from build123d import *

# Parameters (mm, degrees)
SKETCH1_W           = 50
SKETCH1_H           = 32
SKETCH1_R           = 9.5
SKETCH1_R_2         = 1.65
BOSS_EXTRUDE1_DEPTH = 6.35
SKETCH2_R           = 1.65
CUT_EXTRUDE1_DEPTH  = 31.892110643
FILLET1_R           = 4


with BuildPart() as part:
    # Sketch1 → Boss-Extrude1 (new body)
    with BuildSketch(Plane.XY):
        with Locations((0, -1)):
            Rectangle(SKETCH1_W, SKETCH1_H)
        Circle(SKETCH1_R, mode=Mode.SUBTRACT)
        with Locations((-9.192388155, 9.192388155)):
            Circle(SKETCH1_R_2, mode=Mode.SUBTRACT)
        with Locations((9.192388155, 9.192388155)):
            Circle(SKETCH1_R_2, mode=Mode.SUBTRACT)
        with Locations((9.192388155, -9.192388155)):
            Circle(SKETCH1_R_2, mode=Mode.SUBTRACT)
        with Locations((-9.192388155, -9.192388155)):
            Circle(SKETCH1_R_2, mode=Mode.SUBTRACT)
    extrude(amount=BOSS_EXTRUDE1_DEPTH)

    # Sketch2 → Cut-Extrude1 (cut, through all)
    with BuildSketch(Plane.XY.offset(6.35)):
        with Locations((-20, 6)):
            Circle(SKETCH2_R)
        with Locations((-20, -13)):
            Circle(SKETCH2_R)
        with Locations((20, -13)):
            Circle(SKETCH2_R)
        with Locations((20, 6)):
            Circle(SKETCH2_R)
    extrude(amount=-CUT_EXTRUDE1_DEPTH, mode=Mode.SUBTRACT)

    # Fillet1
    fillet1_edges = [part.edges().sort_by_distance(p)[0] for p in [
        (-25, 15, 3.175),
        (25, 15, 3.175),
        (25, -17, 3.175),
        (-25, -17, 3.175),
    ]]
    fillet(fillet1_edges, radius=FILLET1_R)


solid = part.part
For this review, take the finished solid that the model builds, in its own axes (mm). Round coordinates to 2 decimals unless told otherwise and drop trailing zeros. Loops run counter-clockwise (first coordinate to the right, second up) from the corner with the lowest first, then second, coordinate; pieces in that order, holes last. Notation, with made-up numbers: (36.25, 76.5) - (81.25, 76.5) arc R31 cw to (81.25, 111.5) - close; hole circle Ø8 at (83, 26.25). An arc over 180 degrees is marked (long way). One line per question, with ' | ' between items.
Q1. Take a section at B-B (y = 0). Give the boundary of the cut face in (x, z), and give its area (3 significant figures).
Taken from the geometry:
outline: (-25, 0) - (-9.5, 0) - (-9.5, 6.35) - (-25, 6.35) - close; (9.5, 0) - (25, 0) - (25, 6.35) - (9.5, 6.35) - close | area: 197 mm²
Q2. For line 1 along Y through (x, z) = (20, 3); line 2 along Y through (x, z) = (-8, 5.25); line 3 along Y through (x, z) = (19, 2.75), list the stretches that pass through material, from the lowest coordinate up. Write a range as [from, to].
Taken from the geometry:
line 1: y = [-17, -14.65], [-11.35, 4.35], [7.65, 15] | line 2: y = [-17, -10.33], [-8.05, -5.12], [5.12, 8.05], [10.33, 15] | line 3: y = [-17, -14.31], [-11.69, 4.69], [7.31, 15]
Q3. Take a section at D-D (z = 5). State how many separate pieces and enclosed holes the cut face has, and give its area (3 significant figures).
Taken from the geometry:
separate pieces: 1 | enclosed holes: 9 | area: 1,230 mm²
Q4. The part is to be moulded in two halves that separate along X. For faces 1 (the cylindrical face through (7.98, 10.31, 3.13)), 2 (the flat face through (25, -1, 3)), 3 (the flat face through (-25, -1, 3)), say which applies: released by +X, released by -X, zero draft, split by the parting line, or undercut.
Taken from the geometry:
face 1: undercut | face 2: released by +X | face 3: released by -X
Q5. Take a section at A-A (x = 0). Give the boundary of the cut face in (y, z), and give its area (4 significant figures).
Taken from the geometry:
outline: (-17, 0) - (-9.5, 0) - (-9.5, 6.35) - (-17, 6.35) - close; (9.5, 0) - (15, 0) - (15, 6.35) - (9.5, 6.35) - close | area: 82.55 mm²
Q6. Take a section at C-C (x = 20). Give the boundary of the cut face in (y, z).
Taken from the geometry:
outline: (-17, 0) - (-14.65, 0) - (-14.65, 6.35) - (-17, 6.35) - close; (-11.35, 0) - (4.35, 0) - (4.35, 6.35) - (-11.35, 6.35) - close; (7.65, 0) - (15, 0) - (15, 6.35) - (7.65, 6.35) - close
Q7. For pin 1 (2 mm diameter, centred on x = -9.19, y = -9.19, fed in from +Z); pin 2 (8 mm diameter, centred on x = -16, y = -7, fed in from -Z), all flat-tipped, find the tip position at first contact; note any pin that passes through.
Taken from the geometry:
pin 1: passes through | pin 2: stops at z = 0
